Source: CAD feature listing. Evaluate the final solid. Frame: model axes, mm. A direction names the side the tool comes from. Coordinates: 2 decimals unless noted, no trailing zeros. Write each loop counter-clockwise with the first axis right and the second up, starting at its lowest first coordinate (ties: lowest second). Pieces come first, ordered by that corner, then holes. Notation, with made-up numbers: (10.25, 24) -> (33.25, 24) arc R8 ccw to (33.25, 30) -> close; hole circle Ø9 at (43, 49). An arc over 180 degrees is marked (long way). One line per item, written item: value. Start each with the question number.
1. Section query C-C, the plane z = 18.75. Output: boundary loops of the cut face in (x, y), and give its area (3 significant figures).
2. Section query B-B, the plane y = 18.5. Output: boundary loops of the cut face in (x, z), and give its area (3 significant figures).
3. Access query for faces 1 (the flat face through (0, -1, 15)), 2 (the cylindrical face through (0.99, -36.77, 0.36)). Directions: +Z, -Z, +X, -X, +Y, -Y. A direction counts if a zero-diameter tool reaches every point of the face in a straight line with its end or side. Return the directions, or none.
4. First-contact query: P1, Ø1.5, axis at y = -11.5, z = 15.5, coming from the -X side; P2, Ø6.5, axis at y = 39.75, z = 12.5, coming from the +X side. Flat tips, straight axial feed; report the tip coordinate or a pass-through.
5. Section query A-A, the plane x = 1.65. State how many separate pieces and enclosed holes the cut face has, and give its area (3 significant figures).
6. Line query: line 1 (Z direction, x = 1.2, y = -39.75); line 2 (Y direction, x = 0.2, z = 10.5); line 3 (Z direction, x = 0.55, y = -48.25). Output: solid intervals per line, ascending.
Autodesk Inventor part; units mm, degrees
ref_plane "YZ Plane" through (0, 0, 0) normal (1, 0, 0) x (0, 1, 0)
ref_plane "XZ Plane" through (0, 0, 0) normal (0, 1, 0) x (-1, 0, 0)
ref_plane "XY Plane" through (0, 0, 0) normal (0, 0, 1) x (1, 0, 0)
sketch "Sketch1" plane through (0, 0, 0) normal (1, 0, 0) x (0, 1, 0)
  line L0 (-39.75, 25) -> (39.75, 25)
  arc A0 (-39.75, 25) -> (-39.75, 0) centre (-39.75, 12.5) ccw
  arc A1 (39.75, 0) -> (39.75, 25) centre (39.75, 12.5) ccw
  circle A2 centre (39.75, 12.5) radius 3.5
  circle A3 centre (39.75, 21) radius 0.75
  circle A4 centre (48.25, 12.5) radius 0.75
  circle A5 centre (39.75, 4) radius 0.75
  circle A6 centre (31.25, 12.5) radius 0.75
  circle A7 centre (-39.75, 12.5) radius 3.5
  circle A8 centre (-48.25, 12.5) radius 0.75
  circle A9 centre (-39.75, 21) radius 0.75
  circle A10 centre (-31.25, 12.5) radius 0.75
  circle A11 centre (-39.75, 4) radius 0.75
  arc A12 (34.0354, 1.3827) -> (-34.0354, 1.3827) centre (0, -64.8302) ccw
  arc A13 (-39.75, 0) -> (-34.0354, 1.3827) centre (-39.75, 12.5) ccw
  arc A14 (34.0354, 1.3827) -> (39.75, 0) centre (39.75, 12.5) ccw
  point P0 (0, 0)
  point P1 (0, 0)
  dimension "d0" = 79.5
  dimension "d1" = 25
  dimension "d2" = 25
  dimension "d3" = 7
  dimension "d4" = 1.5
  dimension "d5" = 1.5
  dimension "d6" = 1.5
  dimension "d7" = 8.5
  dimension "d8" = 8.5
  dimension "d9" = 8.5
  dimension "d10" = 1.5
  dimension "d11" = 8.5
  dimension "d12" = 7
  dimension "d13" = 1.5
  dimension "d14" = 1.5
  dimension "d15" = 1.5
  dimension "d16" = 1.5
  dimension "d17" = 8.5
  dimension "d18" = 8.5
  dimension "d19" = 8.5
  dimension "d20" = 8.5
extrude "Extrusion1" add sketch "Sketch1" along normal blind 2
properties part number "tibia extrude"
Computed values:
1. outline: (0, -50.58) -> (2, -50.58) -> (2, 50.58) -> (0, 50.58) -> close
1. area: 202 mm²
2. outline: (0, 7.28) -> (2, 7.28) -> (2, 25) -> (0, 25) -> close
2. area: 35.4 mm²
3. face 1: +Z, -Z, -X, +Y, -Y
3. face 2: -Z, +X, -X
4. P1: stops at x = 0
4. P2: passes through
5. separate pieces: 1
5. enclosed holes: 10
5. area: 1,910 mm²
6. line 1: z = 0 to 3.25, 4.75 to 9, 16 to 20.25, 21.75 to 25
6. line 2: y = -52.09 to -42.62, -36.88 to 36.88, 42.62 to 52.09
6. line 3: z = 3.33 to 11.75, 13.25 to 21.67
